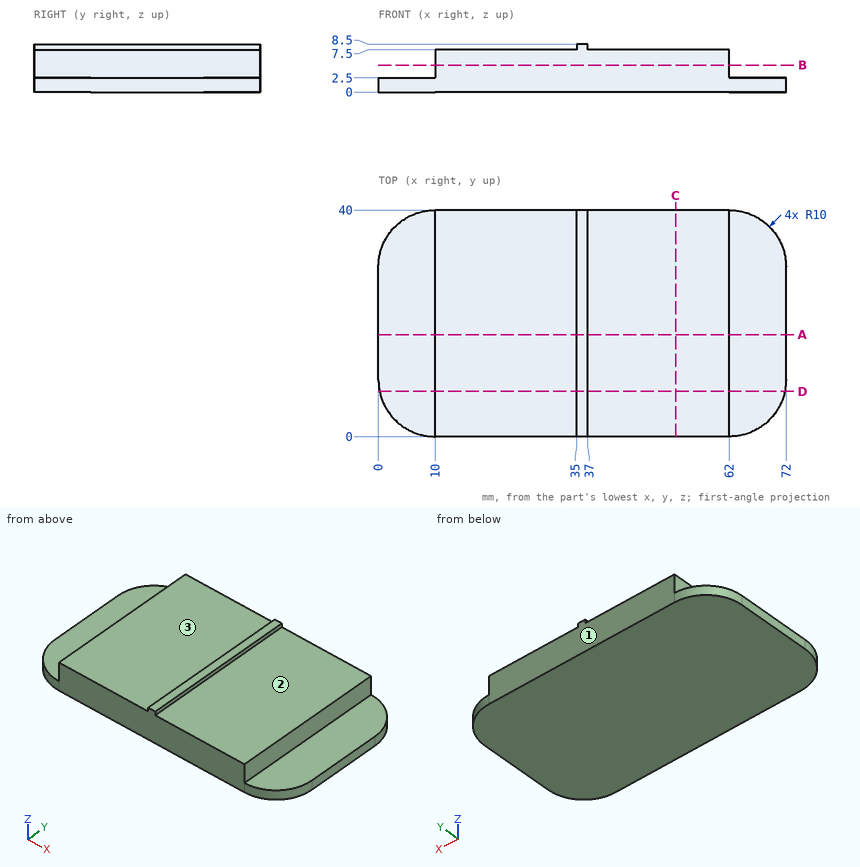
For this review, use the dimensioned drawing (mm, ordinates from the lowest corner) and the shaded views. A direction names the side the tool comes from. Round coordinates to 2 decimals unless told otherwise and drop trailing zeros. Write each loop counter-clockwise with the first axis right and the second up, starting at its lowest first coordinate (ties: lowest second). Pieces come first, ordered by that corner, then holes. Notation, with made-up numbers: M 20.25,-29.5 L 61.25,-29.5 A13 ccw 61.25,-18.5 Z; hole C -2.5,47.25 d1. An arc over 180 degrees is marked long. Use CSV: the item, a comma, the result in double quotes. Start each with the question number.
(1) For line 1 along Z through (x, y) = (16, 34.5); line 2 along X through (y, z) = (8, 4.25), list the stretches that pass through material, from the lowest coordinate up.
(2) We need section C-C, the plane x = 52.5. State the section outline as (y, z) points, then the cut area to 3 significant figures.
(3) We need section D-D, the plane y = 8. State the section outline as (x, z) points.
(4) Clearance check with flat-ended pins moving along their axes: P1, Ø1.5, axis at x = 18, y = 12, coming from the +Z side; P2, Ø4, axis at y = 13, z = 4, coming from the -X side; P3, Ø5, axis at x = 4.5, y = 19.5, coming from the +Z side; P4, Ø1, axis at y = 12.5, z = 6, coming from the -X side. State where each tip first meets the part, or that it passes through.
(5) We need section B-B, the plane z = 4.75. State the section outline as (x, y) points.
(6) We need section A-A, the plane y = 18. State the section outline as (x, z) points, then the cut area to 3 significant figures.
(7) Tool access review of the marked faces 1, 2 and 3: name each direction out of +Z, -Z, +X, -X, +Y, -Y from which nothing blocks a thin tool from reaching the whole face with its end or side.
Findings:
1,line 1,"0 to 7.5"
1,line 2,"10 to 62"
2,outline,"M 0,0 L 40,0 L 40,7.5 L 0,7.5 Z"
2,area,"300 mm^2"
3,outline,"M 0.2,0 L 71.8,0 L 71.8,2.5 L 62,2.5 L 62,7.5 L 37,7.5 L 37,8.5 L 35,8.5 L 35,7.5 L 10,7.5 L 10,2.5 L 0.2,2.5 Z"
4,P1,"z = 7.5"
4,P2,"x = 0"
4,P3,"z = 2.5"
4,P4,"x = 10"
5,outline,"M 10,0 L 62,0 L 62,40 L 10,40 Z"
6,outline,"M 0,0 L 72,0 L 72,2.5 L 62,2.5 L 62,7.5 L 37,7.5 L 37,8.5 L 35,8.5 L 35,7.5 L 10,7.5 L 10,2.5 L 0,2.5 Z"
6,area,"442 mm^2"
7,face 1,"+Z, -Z, +X, -X, +Y"
7,face 2,"+Z, +X, +Y, -Y"
7,face 3,"+Z, -X, +Y, -Y"
